```python
from build123d import *

# Parameters (mm, degrees)
BOSS_EXTRUDE1_DEPTH = 20
SKETCH3_W           = 47.8415773
SKETCH3_H           = 21.769183321
SKETCH3_W_2         = 54.74945498
SKETCH3_H_2         = 26.072393978
BOSS_EXTRUDE2_DEPTH = 20


with BuildPart() as part:
    # Sketch1 → Boss-Extrude1 (new body)
    with BuildSketch(Plane.XY):
        with BuildLine():
            ThreePointArc((-57.85830676, 45.936170213), (-10.937790042, 57.86666983), (35.982726675, 45.936170213))
            Line((35.982726675, 45.936170213), (35.982726675, -85.966261398))
            Line((35.982726675, -85.966261398), (16.952027587, -85.966261398))
            Line((16.952027587, -85.966261398), (16.952027587, 0))
            Line((16.952027587, 0), (-37.187030164, 0))
            Line((-37.187030164, 0), (-37.187030164, -22.639969605))
            Line((-37.187030164, -22.639969605), (-57.85830676, -22.639969605))
            Line((-57.85830676, -22.639969605), (-57.85830676, 0))
            Line((-57.85830676, 0), (-57.85830676, 45.936170213))
        make_face()
    extrude(amount=BOSS_EXTRUDE1_DEPTH)

    # Sketch3 → Boss-Extrude2 (add)
    with BuildSketch(Plane.XY):
        with Locations((-45.869735372, -22.040085901)):
            Rectangle(SKETCH3_W, SKETCH3_H)
        with Locations((27.37472749, -83.170990229)):
            Rectangle(SKETCH3_W_2, SKETCH3_H_2)
    extrude(amount=BOSS_EXTRUDE2_DEPTH)


solid = part.part
```
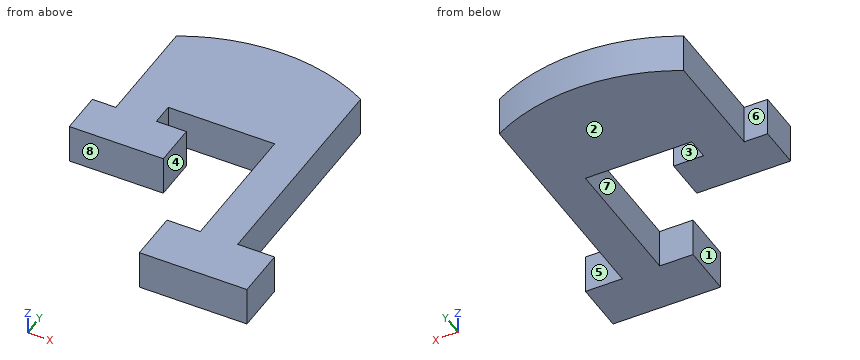
Read the model definition and answer for the solid it produces. Units are mm, in the model's axes. Face numbers are marked on the shaded views. A direction names the side the tool comes from. Give positions to 0.01 mm unless a question says otherwise; leave off trailing zeros. Write each loop counter-clockwise with the first axis right and the second up, starting at its lowest first coordinate (ties: lowest second). Pieces come first, ordered by that corner, then holes. Notation, with made-up numbers: M 65.25,68.5 L 75.25,68.5 A26 cw 75.25,107.5 Z; hole C -39.75,64.5 d9. An arc over 180 degrees is marked long. Put each result on its own line as item: value. Start each with the question number.
1. The part is cut by section B-B, the plane x = 3. Give the vertices of the cut face in (y, z), and give its area (3 significant figures).
2. The part is cut by section D-D, the plane y = -78.5. Give the vertices of the cut face in (x, z), and give its area (3 significant figures).
3. The part is cut by section A-A, the plane y = -29. Give the vertices of the cut face in (x, z), and give its area (3 significant figures).
4. For a pull along X with two mould halves and no side action, classify the marked faces 1, 2 and 3 as released by +X, released by -X, zero draft, split by the parting line, or undercut.
5. Consider line 1 along X through (y, z) = (-19.5, 16.5); line 2 along X through (y, z) = (-4, 12.5); line 3 along Y through (x, z) = (-9, 7.75). Determine where each line is inside the solid, lowest interval first.
6. The part is cut by section C-C, the plane z = 6. Give the vertices of the cut face in (x, y), and give its area (3 significant figures).
7. Which of the six approach directions +Z, -Z, +X, -X, +Y, -Y give full straight-line access (tool end or side, diameter ignored) to the marked faces 4, 5, 6, 7 and 8?
8. Each of these flat-tipped pins is pushed along its axis until it touches: pin 1 Ø12 at (y, z) = (-45.5, 10) entering from -X; pin 2 Ø10 at (y, z) = (-45.5, 3) entering from +X; pin 3 Ø3 at (x, z) = (-49, 8.5) entering from +Y. Where does it stop, or does it pass through?
Final values:
1. outline: M -96.21,0 L -70.13,0 L -70.13,20 L -96.21,20 Z; M 0,0 L 56.87,0 L 56.87,20 L 0,20 Z
1. area: 1,660 mm²
2. outline: M 0,0 L 54.75,0 L 54.75,20 L 0,20 Z
2. area: 1,090 mm²
3. outline: M -69.79,0 L -21.95,0 L -21.95,20 L -69.79,20 Z; M 16.95,0 L 35.98,0 L 35.98,20 L 16.95,20 Z
3. area: 1,340 mm²
4. face 1: released by -X
4. face 2: zero draft
4. face 3: undercut
5. line 1: x = -69.79 to -21.95, 16.95 to 35.98
5. line 2: x = -57.86 to -37.19, 16.95 to 35.98
5. line 3: y = 0 to 57.85
6. outline: M -69.79,-32.92 L -21.95,-32.92 L -21.95,-11.16 L -37.19,-11.16 L -37.19,0 L 16.95,0 L 16.95,-70.13 L 0,-70.13 L 0,-96.21 L 54.75,-96.21 L 54.75,-70.13 L 35.98,-70.13 L 35.98,45.94 A98.23 ccw -57.86,45.94 L -57.86,-11.16 L -69.79,-11.16 Z
6. area: 9,100 mm²
7. face 4: +Z, -Z, -Y
7. face 5: +Z, -Z, +X, +Y
7. face 6: +Z, -Z, -X, +Y
7. face 7: +Z, -Z
7. face 8: +Z, -Z, -X, -Y
8. pin 1: stops at x = 16.95
8. pin 2: stops at x = 35.98
8. pin 3: stops at y = 50.81
